Model file for the job. Use its own axes, mm. Coordinates: 2 decimals unless noted, no trailing zeros. Order: outer loops, then holes, each group sorted by start corner. A loop starts at its lowest first (then second) coordinate and runs counter-clockwise, first axis right, second up. Notation, with made-up numbers: (74, 74) -> (109, 74) arc R24 cw to (109, 95) -> close; hole circle Ø11 at (-34, 11.25). An arc over 180 degrees is marked (long way). Return JSON: item names as keys, results as strings. Group by question number.
1) Flat gauge pins, fed straight in: pin 1 (1 mm diameter, centred on y = -17, z = 0.5, fed in from -X); pin 2 (10 mm diameter, centred on x = 43, y = 31.5, fed in from -Z); pin 3 (1 mm diameter, centred on y = -24.5, z = 1.5, fed in from +X); pin 4 (3.5 mm diameter, centred on x = -52.5, y = 0, fed in from +Z). Where does each tip first touch, or does it go through?
2) Cut at B-B (z = 1.6). Write the cut outline in (x, y), and give its area (3 significant figures).
3) Pull direction Y, two halves, no side cores. Call faces 1 (the cylindrical face through (-54.498, 0.088, 0.986)), 2 (the cylindrical face through (-59.94, 2.64, 1.01)), 3 (the flat face through (-14, -44, 0)): +Y half, -Y half, draft (parallel to the pull), parting line (faces both ways), or undercut.
4) Probe line 1 (Y direction, x = 0, z = 0.5); line 2 (X direction, y = -1, z = 1). List the from-to ranges inside material, lowest first.
5) Cut at A-A (y = 0). Write the cut outline in (x, z).
6) Cut at D-D (y = 52.5). Write the cut outline in (x, z).
from build123d import *

# Parameters (mm, degrees)
SKETCH_1_R          = 75
SKETCH_1_R_2        = 2
SKETCH_1_R_3        = 46
EXTRUDE_1_DEPTH     = 2
SKETCH_2_R          = 1.5
CUT_EXTRUDE_1_DEPTH = 2
SKETCH_4_OUTSIDE_W  = 194.428
SKETCH_4_OUTSIDE_H  = 194.428
SKETCH_4_OUTSIDE_R  = 60
CUT_EXTRUDE_2_DEPTH = 10


with BuildPart() as part:
    # 草图1 → 凸台-拉伸1 (new body)
    with BuildSketch(Plane.XY):
        Circle(SKETCH_1_R)
        with Locations((-52.5, 0)):
            Circle(SKETCH_1_R_2, mode=Mode.SUBTRACT)
        with Locations((0, 52.5)):
            Circle(SKETCH_1_R_2, mode=Mode.SUBTRACT)
        with Locations((52.5, 0)):
            Circle(SKETCH_1_R_2, mode=Mode.SUBTRACT)
        with Locations((0, -52.5)):
            Circle(SKETCH_1_R_2, mode=Mode.SUBTRACT)
        Circle(SKETCH_1_R_3, mode=Mode.SUBTRACT)
    extrude(amount=EXTRUDE_1_DEPTH)

    # 草图2 → 切除-拉伸1 (cut)
    with BuildSketch(Plane.XY.offset(2)):
        with Locations((0, 69)):
            Circle(SKETCH_2_R)
        with Locations((69, 0)):
            Circle(SKETCH_2_R)
        with Locations((0, -69)):
            Circle(SKETCH_2_R)
        with Locations((-69, 0)):
            Circle(SKETCH_2_R)
    extrude(amount=-CUT_EXTRUDE_1_DEPTH, mode=Mode.SUBTRACT)

    # 草图4 outside → 切除-拉伸2 (cut)
    with BuildSketch(Plane.XY.offset(2)):
        Rectangle(SKETCH_4_OUTSIDE_W, SKETCH_4_OUTSIDE_H)
        Circle(SKETCH_4_OUTSIDE_R, mode=Mode.SUBTRACT)
    extrude(amount=-CUT_EXTRUDE_2_DEPTH, mode=Mode.SUBTRACT)


solid = part.part
Answers below:
{
 "1": {"pin 1": "stops at x = -57.69", "pin 2": "stops at z = 0", "pin 3": "stops at x = 54.99", "pin 4": "passes through"},
 "2": {"outline": "circle Ø120 at (0, 0); hole circle Ø4 at (-52.5, 0); hole circle Ø92 at (0, 0); hole circle Ø4 at (0, -52.5); hole circle Ø4 at (0, 52.5); hole circle Ø4 at (52.5, 0)", "area": "4,610 mm^2"},
 "3": {"face 1": "undercut", "face 2": "parting line", "face 3": "draft"},
 "4": {"line 1": "y = -60 to -54.5, -50.5 to -46, 46 to 50.5, 54.5 to 60", "line 2": "x = -59.99 to -54.23, -50.77 to -45.99, 45.99 to 50.77, 54.23 to 59.99"},
 "5": {"outline": "(-60, 0) -> (-54.5, 0) -> (-54.5, 2) -> (-60, 2) -> close; (-50.5, 0) -> (-46, 0) -> (-46, 2) -> (-50.5, 2) -> close; (46, 0) -> (50.5, 0) -> (50.5, 2) -> (46, 2) -> close; (54.5, 0) -> (60, 0) -> (60, 2) -> (54.5, 2) -> close"},
 "6": {"outline": "(-29.05, 0) -> (-2, 0) -> (-2, 2) -> (-29.05, 2) -> close; (2, 0) -> (29.05, 0) -> (29.05, 2) -> (2, 2) -> close"}
}
